Geometry: final body of the model. Coordinates: model frame, mm. A direction names the side the tool comes from. Coordinates: 2 decimals unless noted, no trailing zeros. Order: outer loops, then holes, each group sorted by start corner. A loop starts at its lowest first (then second) coordinate and runs counter-clockwise, first axis right, second up. Notation, with made-up numbers: (63.5, 59.25) -> (121.5, 59.25) arc R30 ccw to (121.5, 82.25) -> close; hole circle Ø7 at (67.5, 71.5). An arc over 180 degrees is marked (long way). Use one line per item in the form item = value.
```python
from build123d import *

# Parameters (mm, degrees)
F0_W     = 381
F0_H     = 63.5
F1_DEPTH = 12.7
F2_W     = 6.35
F2_H     = 12.7
F3_DEPTH = 63.501
F4_W     = 355.6
F4_H     = 6.35
F5_DEPTH = 6.35


with BuildPart() as f1:
    # F0 (on Right) → F1 (new body)
    with BuildSketch(Plane.YZ):
        Rectangle(F0_W, F0_H)
    extrude(amount=F1_DEPTH)

    # F2 (on face) → F3 (cut, through all)
    with BuildSketch(Plane.XY.offset(31.75)):
        with Locations((9.525, 184.15)):
            Rectangle(F2_W, F2_H)
        with Locations((9.525, -184.15)):
            Rectangle(F2_W, F2_H)
    extrude(amount=-F3_DEPTH, mode=Mode.SUBTRACT)

    # F4 (on face) → F5 (cut)
    with BuildSketch(Plane.YZ.offset(12.7)):
        with Locations((0, 22.225)):
            Rectangle(F4_W, F4_H)
        with Locations((0, -22.225)):
            Rectangle(F4_W, F4_H)
    extrude(amount=-F5_DEPTH, mode=Mode.SUBTRACT)


solid = f1.part
```
1) Material intervals for probe 1 along Z at (x, y) = (6.75, -11.5); probe 2 along X at (y, z) = (106.5, -24.5); probe 3 along Y at (x, z) = (11.5, -17), sorted ascending. Write a range as from..to.
Results found:
probe_1 = -31.75..-25.4, -19.05..19.05, 25.4..31.75
probe_2 = 0..6.35
probe_3 = -177.8..177.8
2) Section A-A, the plane x = 9.75. Output: boundary loops of the cut face in (y, z), and give its area (3 significant figures).
Results found:
outline = (-177.8, -31.75) -> (177.8, -31.75) -> (177.8, -25.4) -> (-177.8, -25.4) -> close; (-177.8, -19.05) -> (177.8, -19.05) -> (177.8, 19.05) -> (-177.8, 19.05) -> close; (-177.8, 25.4) -> (177.8, 25.4) -> (177.8, 31.75) -> (-177.8, 31.75) -> close
area = 18,100 mm2
3) Section C-C, the plane y = 54.5. Output: boundary loops of the cut face in (x, z), and give its area (3 significant figures).
Results found:
outline = (0, -31.75) -> (12.7, -31.75) -> (12.7, -25.4) -> (6.35, -25.4) -> (6.35, -19.05) -> (12.7, -19.05) -> (12.7, 19.05) -> (6.35, 19.05) -> (6.35, 25.4) -> (12.7, 25.4) -> (12.7, 31.75) -> (0, 31.75) -> close
area = 726 mm2
4) Access query for faces 1 (the flat face through (9, -177.8, 0)), 2 (the flat face through (10, -2, -19.05)), 3 (the flat face through (9, 177.8, 0)). Directions: +Z, -Z, +X, -X, +Y, -Y. A direction counts if a zero-diameter tool reaches every point of the face in a straight line with its end or side. Return the directions, or none.
Results found:
face_1 = +Z, -Z, +X, -Y
face_2 = +X, +Y, -Y
face_3 = +Z, -Z, +X, +Y
5) Contact query for flat-ended pins moving along their axis: P1, Ø3, axis at x = 10.5, z = -28, coming from the +Y side; P2, Ø1.9, axis at x = 9, z = 2, coming from the -Y side; P3, Ø4, axis at y = 124, z = 17, coming from the -X side. Output: stop coordinate, or through.
Results found:
P1 = 177.8
P2 = -177.8
P3 = 0
6) Section B-B, the plane z = -6. Output: boundary loops of the cut face in (x, y).
Results found:
outline = (0, -190.5) -> (6.35, -190.5) -> (6.35, -177.8) -> (12.7, -177.8) -> (12.7, 177.8) -> (6.35, 177.8) -> (6.35, 190.5) -> (0, 190.5) -> close
7) Pull-direction query (Z, two-part tool) for faces 4 (the flat face through (0, -3, 0)), 5 (the flat face through (6, -3, 31.75)), 6 (the flat face through (10, -2, 19.05)), 7 (the flat face through (10, -2, 25.4)); classes: released by +Z, released by -Z, zero draft, split by the parting line, or undercut.
Results found:
face_4 = zero draft
face_5 = released by +Z
face_6 = undercut
face_7 = undercut
